Autodesk Inventor part; units mm, degrees
ref_plane "YZ Plane" through (0, 0, 0) normal (1, 0, 0) x (0, 1, 0)
ref_plane "XZ Plane" through (0, 0, 0) normal (0, 1, 0) x (-1, 0, 0)
ref_plane "XY Plane" through (0, 0, 0) normal (0, 0, 1) x (1, 0, 0)
sketch "Sketch1" plane through (0, 0, 0) normal (0, 0, 1) x (1, 0, 0)
  circle A0 centre (0, 0) radius 17.5
  circle A1 centre (0, 0) radius 5
  line L0 (0, 5) -> (0, 9)
  arc A2 (0, 9) -> (1.8691, 17.3999) centre (-7.0076, 14.9672) ccw
  arc A3 (1.5, 8.4713) -> (3.471, 17.1523) centre (-7.0076, 14.9672) ccw
  line L1 (1.5, 8.4713) -> (1.5, 4.7697)
  arc A4 (-1.8691, 17.3999) -> (0, 9) centre (7.0076, 14.9672) ccw
  arc A5 (-3.471, 17.1523) -> (-1.5, 8.4713) centre (7.0076, 14.9672) ccw
  line L2 (-1.5, 8.4713) -> (-1.5, 4.7697)
  arc A6 (-6.5864, 5.5347) -> (-13.1189, 11.5821) centre (-16.4658, 1.4148) ccw
  arc A7 (-7.7942, 4.5) -> (-14.1342, 10.3186) centre (-16.4658, 1.4148) ccw
  line L3 (-6.5864, 5.5347) -> (-3.3807, 3.6839)
  line L4 (-4.3301, 2.5) -> (-7.7942, 4.5)
  line L5 (-8.0864, 2.9366) -> (-4.8807, 1.0858)
  arc A8 (-16.5898, 5.5702) -> (-8.0864, 2.9366) centre (-9.4581, 13.5524) ccw
  arc A9 (-16.0033, 7.0813) -> (-7.7942, 4.5) centre (-9.4581, 13.5524) ccw
  arc A10 (-8.0864, -2.9366) -> (-16.5898, -5.5702) centre (-9.4581, -13.5524) ccw
  arc A11 (-7.7942, -4.5) -> (-16.0033, -7.0813) centre (-9.4581, -13.5524) ccw
  line L6 (-8.0864, -2.9366) -> (-4.8807, -1.0858)
  line L7 (-4.3301, -2.5) -> (-7.7942, -4.5)
  line L8 (-6.5864, -5.5347) -> (-3.3807, -3.6839)
  arc A12 (-13.1189, -11.5821) -> (-6.5864, -5.5347) centre (-16.4658, -1.4148) ccw
  arc A13 (-14.1342, -10.3186) -> (-7.7942, -4.5) centre (-16.4658, -1.4148) ccw
  arc A14 (-1.5, -8.4713) -> (-3.471, -17.1523) centre (7.0076, -14.9672) ccw
  arc A15 (0, -9) -> (-1.8691, -17.3999) centre (7.0076, -14.9672) ccw
  line L9 (-1.5, -8.4713) -> (-1.5, -4.7697)
  line L10 (0, -5) -> (0, -9)
  line L11 (1.5, -8.4713) -> (1.5, -4.7697)
  arc A16 (3.471, -17.1523) -> (1.5, -8.4713) centre (-7.0076, -14.9672) ccw
  arc A17 (1.8691, -17.3999) -> (0, -9) centre (-7.0076, -14.9672) ccw
  arc A18 (6.5864, -5.5347) -> (13.1189, -11.5821) centre (16.4658, -1.4148) ccw
  arc A19 (7.7942, -4.5) -> (14.1342, -10.3186) centre (16.4658, -1.4148) ccw
  line L12 (6.5864, -5.5347) -> (3.3807, -3.6839)
  line L13 (4.3301, -2.5) -> (7.7942, -4.5)
  line L14 (8.0864, -2.9366) -> (4.8807, -1.0858)
  arc A20 (16.5898, -5.5702) -> (8.0864, -2.9366) centre (9.4581, -13.5524) ccw
  arc A21 (16.0033, -7.0813) -> (7.7942, -4.5) centre (9.4581, -13.5524) ccw
  arc A22 (8.0864, 2.9366) -> (16.5898, 5.5702) centre (9.4581, 13.5524) ccw
  arc A23 (7.7942, 4.5) -> (16.0033, 7.0813) centre (9.4581, 13.5524) ccw
  line L15 (8.0864, 2.9366) -> (4.8807, 1.0858)
  line L16 (4.3301, 2.5) -> (7.7942, 4.5)
  line L17 (6.5864, 5.5347) -> (3.3807, 3.6839)
  arc A24 (13.1189, 11.5821) -> (6.5864, 5.5347) centre (16.4658, 1.4148) ccw
  arc A25 (14.1342, 10.3186) -> (7.7942, 4.5) centre (16.4658, 1.4148) ccw
  circle A26 centre (0, 0) radius 4
  circle A27 centre (0, 0) radius 16
  point P0 (2.1535, 15.8544)
  point P1 (-2.1535, 15.8544)
  point P2 (15.3247, -4.5992)
  point P3 (15.3247, 4.5992)
  point P4 (3.6793, 15.5712)
  point P5 (11.6454, 10.972)
  point P6 (14.8071, 6.0622)
  point P7 (12.6536, 9.7922)
  point P8 (14.8071, -6.0622)
  point P9 (12.6536, -9.7922)
  point P10 (2.1535, -15.8544)
  point P11 (-2.1535, -15.8544)
  point P12 (11.6454, -10.972)
  point P13 (3.6793, -15.5712)
  point P14 (-3.6793, -15.5712)
  point P15 (-11.6454, -10.972)
  point P16 (-12.6536, -9.7922)
  point P17 (-14.8071, -6.0622)
  point P18 (-15.3247, -4.5992)
  point P19 (-15.3247, 4.5992)
  point P20 (-3.6793, 15.5712)
  point P21 (-11.6454, 10.972)
  point P22 (-14.8071, 6.0622)
  point P23 (-12.6536, 9.7922)
  dimension "d10" = 32
  dimension "d0" = 35
  dimension "d1" = 10
  dimension "d2" = 4
  dimension "d3" = 1.5
  dimension "d4" = 0
  dimension "d7" = 360
  dimension "d9" = 8
extrude "Extrusion1" add sketch "Sketch1" against normal blind 10 contours A0 A20 A27 A22 | A22 A27 A23 A0 | A0 A21 A27 A20 | A23 A27 A25 A0 | A22 L15 A1 L16 A23 A27 | A0 A19 A27 A21 | A27 A21 L13 A1 L14 A20 | A25 A27 A24 A0 | A0 A18 A27 A19 | A24 A27 A3 A0 | A25 L16 A1 L17 A24 A27 | A1 | A0 A16 A27 A18 | A27 A18 L12 A1 L13 A19 | A3 A27 A2 A0 | A0 A17 A27 A16 | A2 A27 A4 A0 | A3 L1 A1 L0 A2 A27 | A0 A15 A27 A17 | A27 A17 L10 A1 L11 A16 | A4 A27 A5 A0 | A0 A14 A27 A15 | A5 A27 A6 A0 | A4 L0 A1 L2 A5 A27 | A0 A12 A27 A14 | A27 A14 L9 A1 L10 A15 | A6 A27 A7 A0 | A0 A13 A27 A12 | A7 A27 A9 A0 | A6 L3 A1 L4 A7 A27 | A0 A11 A27 A13 | A27 A13 L7 A1 L8 A12 | A9 A27 A8 A0 | A1 L5 A8 A27 A9 L4 | A0 A10 A27 A11 | L7 A11 A27 A10 L6 A1 | A8 A27 A10 A0
properties part number "kumandaiç"
Geometry check sheet. Reference: the model listing, model coordinates, mm. Coordinates: 2 decimals unless noted, no trailing zeros. Write each loop counter-clockwise with the first axis right and the second up, starting at its lowest first coordinate (ties: lowest second). Pieces come first, ordered by that corner, then holes. Notation, with made-up numbers: M 20.25,66.25 L 31.25,66.25 A18 ccw 31.25,89.25 Z; hole C 73,26.5 d2. An arc over 180 degrees is marked long. Use one line per item in the form item = value. Start each with the question number.
1) Section check B-B on x = 1. Enter the section's corners in (y, z), and give its area (3 significant figures).
2) Thickness scan on probe 1 along Y at (x, z) = (-11, -9); probe 2 along X at (y, z) = (-6, -8.5); probe 3 along Y at (x, z) = (1, -7). Record the ranges inside material, lowest first. Write a range as from..to.
3) Section check C-C on z = -8.5. State how many separate pieces and enclosed holes the cut face has, and give its area (3 significant figures).
4) Release check for a two-part mould opening along Y. For faces 1 (the cylindrical face through (9.65, -7.6, -4.93)), 2 (the flat face through (1.2, 4, -10)), 3 (the flat face through (-1.5, -7, -5)) record: pulls with the +Y half, pulls with the -Y half, needs draft (parallel to the pull), parting line crosses it, or undercut.
5) Go/stop test with flat-tipped pins: pin 1 Ø1 at (y, z) = (-7, -4.5) entering from -X; pin 2 Ø10 at (x, y) = (-2, -5.5) entering from +Z; pin 3 Ø4 at (y, z) = (-7.5, -7) entering from +X; pin 4 Ø4 at (y, z) = (-6, -4) entering from -X. Record where each tip stops, or that it passes through.
6) Section check A-A on y = 0. Enter the section's corners in (x, z).
Responses:
q1.outline = M -17.47,-10 L -15.97,-10 L -15.97,0 L -17.47,0 Z; M -10.43,-10 L -3.87,-10 L -3.87,0 L -10.43,0 Z; M 3.87,-10 L 10.43,-10 L 10.43,0 L 3.87,0 Z; M 15.97,-10 L 17.47,-10 L 17.47,0 L 15.97,0 Z
q1.area = 161 mm2
q2.probe_1 = -13.61..-11.62, -10.62..-8.82, -4.48..-2.96, 2.96..4.48, 8.82..10.62, 11.62..13.61
q2.probe_2 = -16.44..-14.72, -8.49..-6.79, -1.5..1.5, 6.79..8.49, 14.72..16.44
q2.probe_3 = -17.47..-15.97, -10.43..-3.87, 3.87..10.43, 15.97..17.47
q3.separate_pieces = 1
q3.enclosed_holes = 13
q3.area = 390 mm2
q4.face_1 = undercut
q4.face_2 = needs draft
q4.face_3 = undercut
q5.pin_1 = -16.25
q5.pin_2 = 0
q5.pin_3 = 16.61
q5.pin_4 = -17.04
q6.outline = M -17.5,-10 L -16,-10 L -16,0 L -17.5,0 Z; M -5,-10 L -4,-10 L -4,0 L -5,0 Z; M 4,-10 L 5,-10 L 5,0 L 4,0 Z; M 16,-10 L 17.5,-10 L 17.5,0 L 16,0 Z
